```python
from build123d import *

# Parameters (mm, degrees)
BOSS_EXTRU_1_DEPTH                             = 15
ESQUISSE2_R                                    = 1.2
ENL_V_MAT_EXTRU_1_DEPTH                        = 26.243811123
ESQUISSE3_R                                    = 0.75
ENL_V_MAT_EXTRU_2_DEPTH                        = 20.006577809
ESQUISSE4_R                                    = 1.2
ENL_V_MAT_EXTRU_3_DEPTH                        = 34.470135942
BOSS_EXTRU_2_START                             = 2.3
ESQUISSE5_W                                    = 5.3
ESQUISSE5_H                                    = 9.6
ESQUISSE5_R                                    = 0.75
BOSS_EXTRU_2_DEPTH                             = 2.3
FRAISAGE_POUR_VIS_T_TE_FRAIS_E_M31_D           = 3.2
FRAISAGE_POUR_VIS_T_TE_FRAIS_E_M31_CSINK_D     = 6.3
FRAISAGE_POUR_VIS_T_TE_FRAIS_E_M31_CSINK_ANGLE = 90
ENL_V_MAT_EXTRU_4_DEPTH                        = 2.3
ESQUISSE9_R                                    = 1.2
ENL_V_MAT_EXTRU_5_DEPTH                        = 20.006577853
BOSS_EXTRU_3_DEPTH                             = 16
ESQUISSE11_W                                   = 4
ESQUISSE11_H                                   = 3.2
BOSS_EXTRU_4_DEPTH                             = 10
ESQUISSE14_W                                   = 1.3
ESQUISSE14_H                                   = 4.8
BOSS_EXTRU_5_DEPTH                             = 20
ENL_V_MAT_EXTRU_6_OUTLINE_W                    = 4
ENL_V_MAT_EXTRU_6_OUTLINE_H                    = 9.502069599
ESQUISSE13_R                                   = 1.5
ENL_V_MAT_EXTRU_7_DEPTH                        = 40.865398531


with BuildPart() as part:
    # Esquisse1 → Boss.-Extru.1 (new, symmetric)
    with BuildSketch(Plane(origin=(0, 0, 0), x_dir=(0, 0, -1), z_dir=(1, 0, 0))):
        Polygon((-12.5, -4.8), (-12.5, -8), (0, -8), (0, 8), (-12.5, 8), (-12.5, 4.8), (-8.5, 4.8), (-8.5, -4.8), align=None)
    extrude(amount=BOSS_EXTRU_1_DEPTH, both=True)

    # Esquisse2 → Enlèv. mat.-Extru.1 (cut, through all)
    with BuildSketch(Plane(origin=(0, 8, 0), x_dir=(1, 0, 0), z_dir=(0, 1, 0))):
        with Locations(Location((-7.5, -4, 0), (0, 0, 270))):
            Circle(ESQUISSE2_R)
        with Locations(Location((7.5, -4, 0), (0, 0, 90))):
            Circle(ESQUISSE2_R)
        with Locations(Location((0, -4, 0), (0, 0, 270))):
            Circle(ESQUISSE2_R)
    extrude(amount=-ENL_V_MAT_EXTRU_1_DEPTH, mode=Mode.SUBTRACT)

    # Esquisse3 → Enlèv. mat.-Extru.2 (cut, through all)
    with BuildSketch(Plane.XY.offset(8.5)):
        with Locations((-12, 0)):
            Circle(ESQUISSE3_R)
    extrude(amount=-ENL_V_MAT_EXTRU_2_DEPTH, mode=Mode.SUBTRACT)

    # Esquisse4 → Enlèv. mat.-Extru.3 (cut, through all)
    with BuildSketch(Plane(origin=(15, 0, 0), x_dir=(0, 0, -1), z_dir=(1, 0, 0))):
        with Locations((-4, -4.5)):
            Circle(ESQUISSE4_R)
        with Locations(Location((-4, 4.5, 0), (0, 0, 180))):
            Circle(ESQUISSE4_R)
    extrude(amount=-ENL_V_MAT_EXTRU_3_DEPTH, mode=Mode.SUBTRACT)

    # Esquisse5 → Boss.-Extru.2 (add)
    with BuildSketch(Plane.XY.offset(8.5).offset(BOSS_EXTRU_2_START)):
        with Locations((-12.35, 0)):
            Rectangle(ESQUISSE5_W, ESQUISSE5_H)
        with Locations((-12, 0)):
            Circle(ESQUISSE5_R, mode=Mode.SUBTRACT)
    extrude(amount=-BOSS_EXTRU_2_DEPTH)

    # Fraisage pour vis à tête fraisée M31 (through all)
    with Locations(Plane.XY.offset(8.5)):
        with Locations((0, 0)):
            CounterSinkHole(FRAISAGE_POUR_VIS_T_TE_FRAIS_E_M31_D / 2, FRAISAGE_POUR_VIS_T_TE_FRAIS_E_M31_CSINK_D / 2, counter_sink_angle=FRAISAGE_POUR_VIS_T_TE_FRAIS_E_M31_CSINK_ANGLE)

    # Esquisse8 → Enlèv. mat.-Extru.4 (cut)
    with BuildSketch(Plane(origin=(0, 0, 0), x_dir=(-1, 0, 0), z_dir=(0, 0, -1))):
        Polygon((14.8, 1.616580754), (12, 3.233161507), (9.2, 1.616580754), (9.2, -1.616580754), (12, -3.233161507), (14.8, -1.616580754), align=None)
    extrude(amount=-ENL_V_MAT_EXTRU_4_DEPTH, mode=Mode.SUBTRACT)

    # Esquisse9 → Enlèv. mat.-Extru.5 (cut, through all)
    with BuildSketch(Plane.XY.offset(8.5)):
        with Locations((5, 0)):
            Circle(ESQUISSE9_R)
    extrude(amount=-ENL_V_MAT_EXTRU_5_DEPTH, mode=Mode.SUBTRACT)

    # Esquisse10 → Boss.-Extru.3 (add)
    with BuildSketch(Plane.XZ.offset(8)):
        Polygon((25, 8.5), (-9, 8.5), (-9, 0), (12.5, 0), (24, -11.5), (25, -11.5), align=None)
    extrude(amount=-BOSS_EXTRU_3_DEPTH)

    # Esquisse11 → Boss.-Extru.4 (add)
    with BuildSketch(Plane(origin=(15, 0, 0), x_dir=(0, 0, -1), z_dir=(1, 0, 0))):
        with Locations((-10.5, -6.4)):
            Rectangle(ESQUISSE11_W, ESQUISSE11_H)
        with Locations((-10.5, 6.4)):
            Rectangle(ESQUISSE11_W, ESQUISSE11_H)
    extrude(amount=BOSS_EXTRU_4_DEPTH)

    # Esquisse14 → Boss.-Extru.5 (add)
    with BuildSketch(Plane.XY.offset(8.5)):
        with Locations((25.65, 0)):
            Rectangle(ESQUISSE14_W, ESQUISSE14_H)
    extrude(amount=-BOSS_EXTRU_5_DEPTH)

    # Enlèv. mat.-Extru.6: read off the stored shape, not the designer's step
    # Enlèv. mat.-Extru.6 outline → Enlèv. mat.-Extru.6 (revolve, cut)
    with BuildSketch(Plane.YX.offset(4)):
        with Locations((2, 17.248965201)):
            Rectangle(ENL_V_MAT_EXTRU_6_OUTLINE_W, ENL_V_MAT_EXTRU_6_OUTLINE_H)
    revolve(axis=Axis((0, 0, -4), (1, 0, 0)), mode=Mode.SUBTRACT)

    # Esquisse13 → Enlèv. mat.-Extru.7 (cut, through all)
    with BuildSketch(Plane.ZY.offset(-22)):
        with Locations((-4, 0)):
            Circle(ESQUISSE13_R)
    extrude(amount=-ENL_V_MAT_EXTRU_7_DEPTH, mode=Mode.SUBTRACT)


solid = part.part
```
Check sheet for the modelled part. Datum: model origin and axes. Units: mm. A direction names the side the tool comes from. Give positions to 0.01 mm unless a question says otherwise; leave off trailing zeros. Loops run counter-clockwise (first coordinate to the right, second up) from the corner with the lowest first, then second, coordinate; pieces in that order, holes last. Notation, with made-up numbers: M 20.25,-18 L 61.25,-18 A4 cw 61.25,-13 Z; hole C 80.25,5 d4. An arc over 180 degrees is marked long. Answer as CSV lines item,"result".
Item 1: Sectioned sample at C-C, the plane y = 6.5. Enter the section's corners in (x, z), then the cut area to 3 significant figures.
Reply:
outline,"M -15,0 L 12.5,0 L 24,-11.5 L 25,-11.5 L 25,12.5 L -15,12.5 Z"
area,"578 mm^2"
Item 2: Scan lines: L1, parallel to Y at x = -13.7, z = 4; L2, parallel to Y at x = -12, z = 7; L3, parallel to X at y = -6.5, z = 2.25. Record each from-to range of solid material in increasing order.
Reply:
L1,"-8 to -5.7, -3.3 to 3.3, 5.7 to 8"
L2,"-8 to -0.75, 0.75 to 8"
L3,"-15 to 25"
Item 3: Sectioned sample at A-A, the plane z = -4. Enter the section's corners in (x, y), then the cut area to 3 significant figures.
Reply:
outline,"M 16.5,-8 L 25,-8 L 25,-2.4 L 26.3,-2.4 L 26.3,-1.5 L 22,-1.5 L 22,-4 L 16.5,-4 Z; M 16.5,4 L 22,4 L 22,1.5 L 26.3,1.5 L 26.3,2.4 L 25,2.4 L 25,8 L 16.5,8 Z"
area,"85.3 mm^2"
Item 4: Draft check along Z on faces 1 (the face through (5, -6, 12.5)), 2 (the face through (-11, -1, 2.3)), 3 (the face through (24.12, -0.575, -2.614)), 4 (the face through (25, 5, 1)). Enter one of: pulls with the +Z half, pulls with the -Z half, needs draft (parallel to the pull), parting line crosses it, or undercut.
Reply:
face 1,"pulls with the +Z half"
face 2,"pulls with the -Z half"
face 3,"undercut"
face 4,"needs draft"
Item 5: Depth check by flat-ended pin: pin 1 Ø4 at (x, y) = (-13.5, 1.5) entering from +Z; pin 2 Ø5 at (y, z) = (0, -4) entering from -X; pin 3 Ø3 at (y, z) = (4, 3.5) entering from +X; pin 4 Ø5 at (x, z) = (-0.5, -4.5) entering from -Y. Enter the tip coordinate at first touch or a pass-through.
Reply:
pin 1,"z = 10.8"
pin 2,"x = 22"
pin 3,"x = 25"
pin 4,"through"
Item 6: Sectioned sample at B-B, the plane z = 4. Enter the section's corners in (x, y), then the cut area to 3 significant figures.
Reply:
outline,"M -15,-8 L 25,-8 L 25,-2.4 L 26.3,-2.4 L 26.3,2.4 L 25,2.4 L 25,8 L -15,8 L -15,5.7 L -9,5.7 L -9,3.3 L -15,3.3 L -15,-3.3 L -9,-3.3 L -9,-5.7 L -15,-5.7 Z; hole C -12,0 d1.5"
area,"616 mm^2"
Item 7: Sectioned sample at D-D, the plane x = 0. Enter the section's corners in (y, z), then the cut area to 3 significant figures.
Reply:
outline,"M -8,0 L 8,0 L 8,12.5 L 4.8,12.5 L 4.8,8.5 L -4.8,8.5 L -4.8,12.5 L -8,12.5 Z"
area,"162 mm^2"
Item 8: Set-up check for faces 5 (the face through (-11.96, -4.45, 5.2)), 6 (the face through (26, -2.4, -1)), 7 (the face through (-9.2, 0, 1)), 8 (the face through (-13, 0, 10.8)): record each of +Z, -Z, +X, -X, +Y, -Y from which the full face is reachable in a straight line by a thin tool's end or side.
Reply:
face 5,"-X"
face 6,"+Z, -Z, +X, -Y"
face 7,"-Z"
face 8,"+Z, +X, -X"
